from build123d import *

# Parameters (mm, degrees)
SKETCH1_W           = 59.5
SKETCH1_H           = 4
SKETCH1_W_2         = 4
SKETCH1_W_3         = 44
BOSS_EXTRUDE1_DEPTH = 123


with BuildPart() as part:
    # Sketch1 → Boss-Extrude1 (new body)
    with BuildSketch(Plane(origin=(0, 0, 0), x_dir=(1, 0, 0), z_dir=(0, 1, 0))):
        with Locations((-77.75, 23)):
            Rectangle(SKETCH1_W, SKETCH1_H)
        with Locations((-46, 23)):
            Rectangle(SKETCH1_W_2, SKETCH1_H)
        Polygon((-48, 0), (-44, 0), (-44, 4), (-44, 21), (-48, 21), align=None)
        with Locations((-22, 2)):
            Rectangle(SKETCH1_W_3, SKETCH1_H)
        Polygon((-44, 4), (0, 4), (0, 25), (-44, 25), (-44, 21), align=None)
    extrude(amount=BOSS_EXTRUDE1_DEPTH)


solid = part.part
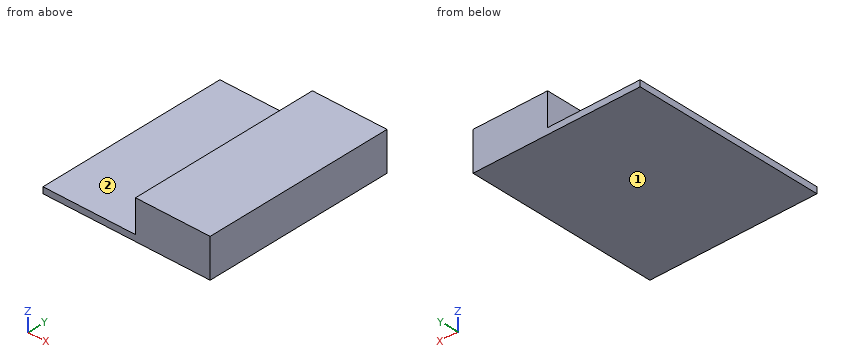
Read the model definition and answer for the solid it produces. Units are mm, in the model's axes. Face numbers are marked on the shaded views. A direction names the side the tool comes from. Round coordinates to 2 decimals unless told otherwise and drop trailing zeros. Loops run counter-clockwise (first coordinate to the right, second up) from the corner with the lowest first, then second, coordinate; pieces in that order, holes last.
Q1. Section B-B on x = -87 is taken. Write down the section's boundary in (y, z), and give its area (3 significant figures).
Q2. Which of the six approach directions +Z, -Z, +X, -X, +Y, -Y give full straight-line access (tool end or side, diameter ignored) to the marked faces 1 and 2?
Q3. Consider probe 1 along X at (y, z) = (36.5, -9.75); probe 2 along Z at (x, y) = (-53, 71). Determine where each line is inside the solid, lowest interval first.
Q4. Section C-C on z = -9 is taken. Write down the section's boundary in (x, y).
Q5. Section A-A on y = 64 is taken. Write down the section's boundary in (x, z), and give its area (3 significant figures).
Q6. Each of these flat-tipped pins is pushed along its axis until it touches: pin 1 (8 mm diameter, centred on y = 97.5, z = -21, fed in from +X); pin 2 (18 mm diameter, centred on x = -64.5, y = 74, fed in from +Z); pin 3 (10.5 mm diameter, centred on y = 50.5, z = -9, fed in from -X). Where does it stop, or does it pass through?
Output:
1. outline: (0, -25) - (123, -25) - (123, -21) - (0, -21) - close
1. area: 492 mm2
2. face 1: -Z, +X, -X, +Y, -Y
2. face 2: +Z, -X, +Y, -Y
3. probe 1: x = -48 to 0
3. probe 2: z = -25 to -21
4. outline: (-48, 0) - (0, 0) - (0, 123) - (-48, 123) - close
5. outline: (-107.5, -25) - (0, -25) - (0, 0) - (-48, 0) - (-48, -21) - (-107.5, -21) - close
5. area: 1,440 mm2
6. pin 1: stops at x = 0
6. pin 2: stops at z = -21
6. pin 3: stops at x = -48
